Build history of the part. All positions in model axes, mm. Face numbers are marked on the shaded views. A direction names the side the tool comes from. Give positions to 0.01 mm unless a question says otherwise; leave off trailing zeros. Order: outer loops, then holes, each group sorted by start corner. A loop starts at its lowest first (then second) coordinate and runs counter-clockwise, first axis right, second up. Notation, with made-up numbers: (5.5, 2.25) - (57.5, 2.25) arc R33 cw to (57.5, 41.25) - close; hole circle Ø11 at (32.25, -22). An arc over 180 degrees is marked (long way). Write each question's results on one line, items separated by ' | '. Start each with the question number.
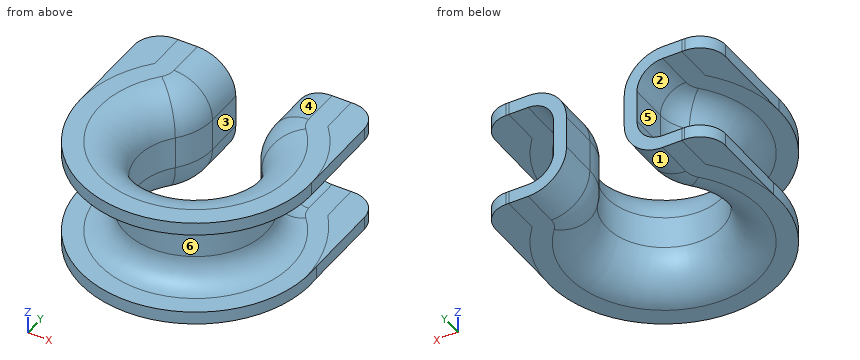
from build123d import *

# Parameters (mm, degrees)
BOSS_EXTRUDE1_START = -8.508956
BOSS_EXTRUDE1_DEPTH = 2
BOSS_EXTRUDE2_START = 8.508956
BOSS_EXTRUDE2_DEPTH = 2
FILLET1_R           = 4


with BuildPart() as part:
    # Sweep2: sweep along a path in Sketch2
    with BuildLine(Plane.XY) as sweep2_path:
        Line((-4.5, 18), (-4.5, 11.9058809))
        ThreePointArc((-4.5, 11.9058809), (-5.08127088, 8.723900384), (-6.75, 5.95294045))
        ThreePointArc((-6.75, 5.95294045), (0, -9), (6.75, 5.95294045))
        ThreePointArc((6.75, 5.95294045), (5.08127088, 8.723900384), (4.5, 11.9058809))
        Line((4.5, 11.9058809), (4.5, 18))
    # Sketch5 → Sweep2 (sweep)
    with BuildSketch(Plane(origin=(0, 0, 0), x_dir=(0, 0, -1), z_dir=(1, 0, 0))):
        with BuildLine():
            Line((-2.508956399, -9), (2.508956399, -9))
            ThreePointArc((2.508956399, -9), (6.751597087, -10.757359313), (8.508956399, -15))
            Line((8.508956399, -15), (8.508956399, -18))
            Line((8.508956399, -18), (6.508956399, -18))
            Line((6.508956399, -18), (6.508956399, -15))
            ThreePointArc((6.508956399, -15), (5.337383524, -12.171572875), (2.508956399, -11))
            Line((2.508956399, -11), (-2.508956399, -11))
            ThreePointArc((-2.508956399, -11), (-5.337383524, -12.171572875), (-6.508956399, -15))
            Line((-6.508956399, -15), (-6.508956399, -18))
            Line((-6.508956399, -18), (-8.508956399, -18))
            Line((-8.508956399, -18), (-8.508956399, -15))
            ThreePointArc((-8.508956399, -15), (-6.751597087, -10.757359313), (-2.508956399, -9))
        make_face()
    sweep(path=sweep2_path.line)

    # Sketch7 → Boss-Extrude1 (add)
    with BuildSketch(Plane.XY.offset(BOSS_EXTRUDE1_START)):
        with BuildLine():
            Line((17.940697807, -1.45991856), (17.940697807, 18))
            Line((17.940697807, 18), (13.5, 18))
            Line((13.5, 18), (13.5, 11.9058809))
            ThreePointArc((13.5, 11.9058809), (16.801469128, 5.58217616), (17.940697807, -1.45991856))
        make_face()
        with BuildLine():
            Line((-13.5, 18), (-13.5, 11.9058809))
            ThreePointArc((-13.5, 11.9058809), (-16.801469128, 5.58217616), (-17.940697807, -1.45991856))
            Line((-17.940697807, -1.45991856), (-17.940697807, 18))
            Line((-17.940697807, 18), (-13.5, 18))
        make_face()
    extrude(amount=BOSS_EXTRUDE1_DEPTH)

    # Sketch9 → Boss-Extrude2 (add)
    with BuildSketch(Plane.XY.offset(BOSS_EXTRUDE2_START)):
        with BuildLine():
            Line((18, 0), (17.940697807, 18))
            Line((17.940697807, 18), (13.5, 18))
            Line((13.5, 18), (13.5, 11.9058809))
            ThreePointArc((13.5, 11.9058809), (16.827327901, 6.360132122), (18, 0))
        make_face()
        with BuildLine():
            Line((-13.5, 18), (-13.5, 11.9058809))
            ThreePointArc((-13.5, 11.9058809), (-16.827327901, 6.360132122), (-18, 0))
            Line((-18, 0), (-17.940697807, 18))
            Line((-17.940697807, 18), (-13.5, 18))
        make_face()
    extrude(amount=-BOSS_EXTRUDE2_DEPTH)

    # Fillet1
    fillet1_edges = [part.edges().sort_by_distance(p)[0] for p in [
        (17.940697807, 18, 7.508956),
        (17.940697807, 18, -7.508956),
        (-17.940697807, 18, 7.508956),
        (-17.940697807, 18, -7.508956),
    ]]
    fillet(fillet1_edges, radius=FILLET1_R)


solid = part.part
Item 1: Two-plate mould, pull along X, no slides. Class the marked faces 4, 5 and 6: +X half, -X half, draft (parallel to the pull), parting line (faces both ways), or undercut.
Item 2: Flat gauge pins, fed straight in: pin 1 Ø0.6 at (y, z) = (8, -8) entering from +X; pin 2 Ø3 at (y, z) = (12.5, 5.5) entering from -X; pin 3 Ø6 at (y, z) = (-4.5, 3) entering from +X; pin 4 Ø8 at (x, z) = (-14, 4.5) entering from +Y. Where does each tip first touch, or does it go through?
Item 3: Probe line 1 along Z through (x, y) = (12, 16); line 2 along X through (y, z) = (0, 0.25); line 3 along Z through (x, y) = (-9.5, -7.5). List the from-to ranges inside material, lowest first. Write a range as from..to.
Item 4: Which spindle directions (+Z, -Z, +X, -X, +Y, -Y) get a long thin tool onto all of the face, cutting with end or side? Do the marked faces 1, 2 and 3. Say none if no direction does.
Item 5: Cut at B-B, the plane x = 0. List the corners of the cut face in (y, z), then the cut area to 3 significant figures.
Item 6: Cut at A-A, the plane z = 1.75. List the corners of the cut face in (x, y), then the cut area to 3 significant figures.
Values found:
1) face 4: undercut | face 5: -X half | face 6: parting line
2) pin 1: stops at x = 17.94 | pin 2: stops at x = -17.96 | pin 3: stops at x = 12.34 | pin 4: stops at y = 18
3) line 1: z = -8.51..-6.51, 6.51..8.51 | line 2: x = -11..-9, 9..11 | line 3: z = -7.76..-5.27, 5.27..7.76
4) face 1: -Z, +Y | face 2: -X, +Y | face 3: +Z, -Z, +Y
5) outline: (-18, -8.51) - (-15, -8.51) arc R6 ccw to (-9, -2.51) - (-9, 2.51) arc R6 ccw to (-15, 8.51) - (-18, 8.51) - (-18, 6.51) - (-15, 6.51) arc R4 cw to (-11, 2.51) - (-11, -2.51) arc R4 cw to (-15, -6.51) - (-18, -6.51) - close | area: 53.5 mm2
6) outline: (-8.25, 7.28) arc R11 ccw (long way) to (8.25, 7.28) arc R7 cw to (6.5, 11.91) - (6.5, 18) - (4.5, 18) - (4.5, 11.91) arc R9 ccw to (6.75, 5.95) arc R9 cw (long way) to (-6.75, 5.95) arc R9 ccw to (-4.5, 11.91) - (-4.5, 18) - (-6.5, 18) - (-6.5, 11.91) arc R7 cw to start | area: 139 mm2
